Design review of the part built by this model. Coordinates are the model's own, in mm. A direction names the side the tool comes from. Coordinates: 2 decimals unless noted, no trailing zeros. Write each loop counter-clockwise with the first axis right and the second up, starting at its lowest first coordinate (ties: lowest second). Pieces come first, ordered by that corner, then holes. Notation, with made-up numbers: (67.25, 12) - (110.25, 12) arc R26 cw to (110.25, 28) - close; hole circle Ø1 at (2.25, 44). An arc over 180 degrees is marked (long way). One line per item, written item: value.
from build123d import *

# Parameters (mm, degrees)
SKETCH_1_R          = 30
EXTRUDE_1_DEPTH     = 15
SKETCH_2_R          = 25
CUT_EXTRUDE_1_DEPTH = 12
SKETCH_3_R          = 4
CUT_EXTRUDE_2_DEPTH = 61


with BuildPart() as part:
    # 草图1 → 凸台-拉伸1 (new body)
    with BuildSketch(Plane(origin=(0, 0, 0), x_dir=(1, 0, 0), z_dir=(0, 1, 0))):
        with Locations(Location((0, 0, 0), (0, 0, 270))):
            Circle(SKETCH_1_R)
    extrude(amount=EXTRUDE_1_DEPTH)

    # 草图2 → 切除-拉伸1 (cut)
    with BuildSketch(Plane(origin=(0, 0, 0), x_dir=(1, 0, 0), z_dir=(0, 1, 0))):
        with Locations(Location((0, 0, 0), (0, 0, 270))):
            Circle(SKETCH_2_R)
    extrude(amount=CUT_EXTRUDE_1_DEPTH, mode=Mode.SUBTRACT)

    # 草图3 → 切除-拉伸2 (cut, symmetric)
    with BuildSketch(Plane(origin=(0, 15, 0), x_dir=(1, 0, 0), z_dir=(0, 1, 0))):
        with Locations(Location((0, 0, 0), (0, 0, 270))):
            Circle(SKETCH_3_R)
    extrude(amount=CUT_EXTRUDE_2_DEPTH, both=True, mode=Mode.SUBTRACT)


solid = part.part
1. Insertion check: pin 1 Ø4 at (y, z) = (9, 0) entering from +X; pin 2 Ø6.5 at (x, z) = (0, 0) entering from +Y; pin 3 Ø2 at (x, y) = (-23, 2) entering from -Z; pin 4 Ø1.5 at (x, y) = (-18, 2) entering from -Z. Each pin has a flat end and moves straight along its axis. Give the tip position at first contact, or say it passes through.
Answer block:
pin 1: stops at x = 30
pin 2: passes through
pin 3: stops at z = -20.4
pin 4: stops at z = -24.54
2. Wall thickness on line 1 along X through (y, z) = (14.25, 0); line 2 along X through (y, z) = (6, 0); line 3 along Y through (x, z) = (-11, -1): over which ranges is each line inside the solid? List them lowest first.
Answer block:
line 1: x = -30 to -4, 4 to 30
line 2: x = -30 to -25, 25 to 30
line 3: y = 12 to 15
3. For faces 1 (the face through (7.509, 5.916, 23.846)), 2 (the face through (25, 0, -7)), list the 3-axis set-ups (+Z, -Z, +X, -X, +Y, -Y) from which the entire face can be reached by the end or side of a thin tool; tool diameter is ignored.
Answer block:
face 1: -Y
face 2: +Z, -Z, +X, -X, -Y
4. Mouldability with a two-part tool opening along Z and no side actions: class faces 3 (the face through (0, 15, 6)), 4 (the face through (1.32, 7.4, -29.97)), 5 (the face through (-3.905, 13.521, -0.867)) as released by +Z, released by -Z, zero draft, split by the parting line, or undercut.
Answer block:
face 3: zero draft
face 4: split by the parting line
face 5: undercut
5. Consider section C-C, the plane x = 24. Write out the cut boundary in (y, z), then the cut area to 3 significant figures.
Answer block:
outline: (0, -18) - (15, -18) - (15, 18) - (0, 18) - (0, 7) - (12, 7) - (12, -7) - (0, -7) - close
area: 372 mm^2
6. Consider section D-D, the plane y = 9.75. Write out the cut boundary in (x, z), then the cut area to 3 significant figures.
Answer block:
outline: circle Ø60 at (0, 0); hole circle Ø50 at (0, 0)
area: 864 mm^2
7. Consider section A-A, the plane z = 0. Write out the cut boundary in (x, y).
Answer block:
outline: (-30, 0) - (-25, 0) - (-25, 12) - (-4, 12) - (-4, 15) - (-30, 15) - close; (4, 12) - (25, 12) - (25, 0) - (30, 0) - (30, 15) - (4, 15) - close
8. Consider section B-B, the plane x = 0. Write out the cut boundary in (y, z).
Answer block:
outline: (0, -30) - (15, -30) - (15, -4) - (12, -4) - (12, -25) - (0, -25) - close; (0, 25) - (12, 25) - (12, 4) - (15, 4) - (15, 30) - (0, 30) - close
